The model under review builds one solid part; all positions refer to its coordinate system, in mm. A direction names the side the tool comes from. Round coordinates to 2 decimals unless told otherwise and drop trailing zeros. Order: outer loops, then holes, each group sorted by start corner. A loop starts at its lowest first (then second) coordinate and runs counter-clockwise, first axis right, second up. Notation, with made-up numbers: (-31.5, 51.25) -> (-22.5, 51.25) arc R16 ccw to (-22.5, 68.25) -> close; hole circle Ø6 at (40.25, 19). An arc over 180 degrees is marked (long way). Return JSON: item names as keys, results as strings. Group by question number.
from build123d import *

# Parameters (mm, degrees)
PAD125_DEPTH            = 10
SKETCH264_R             = 2.75
POCKET112_DEPTH         = 41.501
SKETCH265_R             = 2.1
POCKET113_DEPTH         = 16
POCKET114_DEPTH         = 108.4688754286
POCKET114_DEPTH_BACK    = 125.0688754286
SKETCH_R                = 3.25
POCKET_DEPTH            = 34.901
BODY089_PITCH_ANGLE     = -90
BODY089_PLACEMENT_ANGLE = -180


with BuildPart() as part:
    # Sketch263 → Pad125 (new body, symmetric)
    with BuildSketch(Plane.YZ):
        with BuildLine():
            Line((-16.6, 41.5), (-16.6, 39.5))
            ThreePointArc((-16.6, 39.5), (-16.0142135624, 38.0857864376), (-14.6, 37.5))
            Line((-14.6, 37.5), (-8.6, 37.5))
            ThreePointArc((-6.6, 35.5), (-7.1857864376, 36.9142135624), (-8.6, 37.5))
            Line((-6.6, 35.5), (-6.6, -4.1))
            ThreePointArc((-6.6, -4.1), (-6.0142135624, -5.5142135624), (-4.6, -6.1))
            Line((-4.6, -6.1), (0, -6.1))
            Line((0, -6.1), (0, -0.1))
            Line((0, -0.1), (-4.6, -0.1))
            Line((-4.6, -0.1), (-4.6, 6.6))
            Line((-4.6, 6.6), (0, 6.6))
            Line((0, 6.6), (0, 41.5))
            Line((0, 41.5), (-16.6, 41.5))
        make_face()
    extrude(amount=PAD125_DEPTH, both=True)

    # Sketch264 → Pocket112 (cut, through all)
    with BuildSketch(Plane(origin=(0, 0, 0), x_dir=(-1, 0, 0), z_dir=(0, 0, -1))):
        with Locations((0, -11.6)):
            Circle(SKETCH264_R)
    extrude(amount=-POCKET112_DEPTH, mode=Mode.SUBTRACT)

    # Sketch265 (on Face7 of Pocket112) → Pocket113 (cut)
    with BuildSketch(Plane.YX.offset(0.1)):
        with Locations((0, -3.5)):
            Circle(SKETCH265_R)
    extrude(amount=POCKET113_DEPTH, mode=Mode.SUBTRACT)

    # Sketch266 → Pocket114 (cut, two sides)
    with BuildSketch(Plane.XZ) as pocket114_sk:
        Polygon((10, -6.1), (10, 35.5), (2, -6.1), align=None)
        Polygon((-8, 35), (4.5, 22.5), (-8, 10), align=None)
    extrude(amount=-POCKET114_DEPTH, mode=Mode.SUBTRACT)
    extrude(pocket114_sk.sketch, amount=POCKET114_DEPTH_BACK, mode=Mode.SUBTRACT)

    # Mirrored011: part across XZ


with BuildPart() as part_1:
    add(part.part)
    add(part.part.mirror(Plane.XZ))

    # Sketch (on Face24 of Mirrored011) → Pocket (cut, through all)
    with BuildSketch(Plane.YX.offset(-6.6)):
        with Locations((0, -3.5)):
            Circle(SKETCH_R)
    extrude(amount=-POCKET_DEPTH, mode=Mode.SUBTRACT)


with BuildPart() as part_2:
    # Body089 pitch: moved
    add(part_1.part.rotate(Axis((0, 0, 0), (0, 1, 0)), BODY089_PITCH_ANGLE))


with BuildPart() as part_3:
    # Body089 placement: moved
    add(part_2.part.moved(Location((0, 0, 218))).rotate(Axis((0, 0, 218), (0, 0, 1)), BODY089_PLACEMENT_ANGLE))


solid = part_3.part
Item 1: Wall thickness on line 1 along Y through (x, z) = (38.85, 218); line 2 along Y through (x, z) = (10.5, 214.5); line 3 along Y through (x, z) = (38.5, 218): over which ranges is each line inside the solid? List them lowest first.
Item 2: For faces 1 (the face through (37.5, 9.6, 220.4)), 2 (the face through (6.6, 0, 219)), 3 (the face through (22, 0, 210)), 4 (the face through (37.5, -9.6, 220.4)), list the 3-axis set-ups (+Z, -Z, +X, -X, +Y, -Y) from which the entire face can be reached by the end or side of a thin tool; tool diameter is ignored.
Item 3: Insertion check: pin 1 Ø1.5 at (x, y) = (2.5, -1) entering from -Z; pin 2 Ø3.5 at (x, z) = (3, 214.5) entering from -Y; pin 3 Ø10 at (x, z) = (23, 222) entering from +Y; pin 4 Ø1.5 at (y, z) = (-9.5, 219) entering from -X. Each pin has a flat end and moves straight along its axis. Give the tip position at first contact, or say it passes through.
Item 4: Consider section A-A on z = 221.75. State the section outline as (x, y) points.
Item 5: Consider section B-B on y = -11.6. State the section outline as (x, z) points, plus the area to 3 significant figures.
Item 6: Consider section C-C on x = 17. State the section outline as (y, z) points, plus the area to 3 significant figures.
Item 7: The part is to be moulded in two halves that separate along Y. For faces 5 (the face through (-0.1, 2, 213)), 6 (the face through (-5.5, -6.03, 214.28)), 7 (the face through (-6.1, -2.1, 215.4)), say which applies: +Y half, -Y half, draft (parallel to the pull), parting line (faces both ways), or undercut.
Item 8: Consider section D-D on y = -1.5. State the section outline as (x, z) points.
Values:
{
 "1": {"line 1": "-16.49 to -14.35, -8.85 to 8.85, 14.35 to 16.49", "line 2": "-6.6 to -3.25, 3.25 to 6.6", "line 3": "-16.33 to -14.35, -8.85 to 8.85, 14.35 to 16.33"},
 "2": {"face 1": "+Z, -Z, -X, +Y", "face 2": "+Z, -Z", "face 3": "+Y, -Y", "face 4": "+Z, -Z, -X, -Y"},
 "3": {"pin 1": "through", "pin 2": "y = -6.6", "pin 3": "y = 6.6", "pin 4": "x = 37.5"},
 "4": {"outline": "(3, -6.6) -> (21.75, -6.6) -> (21.75, 6.6) -> (3, 6.6) -> (3, 4.6) -> (6.6, 4.6) -> (6.6, -4.6) -> (3, -4.6) -> close; (23.25, -6.6) -> (35.5, -6.6) arc R2 cw to (37.5, -8.6) -> (37.5, -14.6) arc R2 ccw to (39.5, -16.6) -> (41.5, -16.6) -> (41.5, 16.6) -> (39.5, 16.6) arc R2 ccw to (37.5, 14.6) -> (37.5, 8.6) arc R2 cw to (35.5, 6.6) -> (23.25, 6.6) -> close"},
 "5": {"outline": "(37.5, 208) -> (41.5, 208) -> (41.5, 215.25) -> (37.5, 215.25) -> close; (37.5, 220.75) -> (41.5, 220.75) -> (41.5, 228) -> (37.5, 228) -> close", "area": "58.0 mm^2"},
 "6": {"outline": "(-6.6, 208) -> (6.6, 208) -> (6.6, 210) -> (-6.6, 210) -> close; (-6.6, 217) -> (-2.08, 217) arc R3.25 cw to (2.08, 217) -> (6.6, 217) -> (6.6, 224.44) -> (-6.6, 224.44) -> close", "area": "123 mm^2"},
 "7": {"face 5": "undercut", "face 6": "-Y half", "face 7": "draft"},
 "8": {"outline": "(-6.1, 208) -> (-0.1, 208) -> (-0.1, 213.03) -> (-6.1, 213.03) -> close; (-6.1, 215.97) -> (-0.1, 215.97) -> (-0.1, 221.15) -> (-6.1, 220) -> close; (6.6, 208) -> (41.5, 208) -> (41.5, 211.62) -> (33.38, 211.62) -> (35, 210) -> (10, 210) -> (11.62, 211.62) -> (6.6, 211.62) -> close; (6.6, 217.38) -> (17.38, 217.38) -> (22.5, 222.5) -> (27.62, 217.38) -> (41.5, 217.38) -> (41.5, 228) -> (35.5, 228) -> (6.6, 222.44) -> close"}
}
